Input: part model. Units: mm. Frame: model coordinates. A direction names the side the tool comes from. Give positions to 0.01 mm unless a question says otherwise; leave off trailing zeros. Write each loop counter-clockwise with the first axis right and the second up, starting at its lowest first coordinate (ties: lowest second). Pieces come first, ordered by that corner, then holes.
```python
from build123d import *

# Parameters (mm, degrees)
SKETCH1_W           = 50
SKETCH1_H           = 58
BOSS_EXTRUDE1_DEPTH = 3
SKETCH2_W           = 50
SKETCH2_H           = 3
BOSS_EXTRUDE2_DEPTH = 20
SKETCH6_R           = 3
BOSS_EXTRUDE3_DEPTH = 25
SKETCH7_R           = 6
CUT_EXTRUDE2_DEPTH  = 24
SKETCH9_R           = 1.9
CUT_EXTRUDE3_DEPTH  = 4
SKETCH10_R          = 1.25
CUT_EXTRUDE4_DEPTH  = 10
BOSS_EXTRUDE4_REACH = 31.5
SKETCH11_R          = 4.5
SKETCH12_R          = 3
SKETCH12_R_2        = 2.25
CUT_EXTRUDE5_DEPTH  = 1


with BuildPart() as part:
    # Sketch1 → Boss-Extrude1 (new body)
    with BuildSketch(Plane.XY):
        with Locations((-30.619684785, 7.512687188)):
            Rectangle(SKETCH1_W, SKETCH1_H)
    extrude(amount=BOSS_EXTRUDE1_DEPTH)

    # Sketch2 → Boss-Extrude2 (add)
    with BuildSketch(Plane(origin=(0, 0, 0), x_dir=(-1, 0, 0), z_dir=(0, 0, -1))):
        with Locations((30.619684785, -19.987312812)):
            Rectangle(SKETCH2_W, SKETCH2_H)
    extrude(amount=BOSS_EXTRUDE2_DEPTH)

    # Sketch6 → Boss-Extrude3 (add)
    with BuildSketch(Plane.XY.offset(3)):
        with Locations((-30.619684785, -1.487312812)):
            Circle(SKETCH6_R)
    extrude(amount=BOSS_EXTRUDE3_DEPTH)

    # Sketch7 → Cut-Extrude2 (cut, through all)
    with BuildSketch(Plane.XY.offset(3)):
        with Locations((-30.619684785, 21.012687188)):
            Circle(SKETCH7_R)
    extrude(amount=-CUT_EXTRUDE2_DEPTH, mode=Mode.SUBTRACT)

    # Sketch9 → Cut-Extrude3 (cut, through all)
    with BuildSketch(Plane(origin=(0, -18.487312812, 0), x_dir=(1, 0, 0), z_dir=(0, 1, 0))):
        with Locations((-18.119684785, 10)):
            Circle(SKETCH9_R)
        with Locations((-43.119684785, 10)):
            Circle(SKETCH9_R)
    extrude(amount=-CUT_EXTRUDE3_DEPTH, mode=Mode.SUBTRACT)

    # Sketch10 → Cut-Extrude4 (cut)
    with BuildSketch(Plane.XY.offset(3)):
        with Locations((-40.145964226, 26.512687188)):
            Circle(SKETCH10_R)
        with Locations((-21.093405343, 26.512687188)):
            Circle(SKETCH10_R)
        with Locations((-30.619684785, 10.012687188)):
            Circle(SKETCH10_R)
    extrude(amount=-CUT_EXTRUDE4_DEPTH, mode=Mode.SUBTRACT)

    # Sketch11 → Boss-Extrude4 (add, up to next)
    with BuildSketch(Plane.XY.offset(9.5), mode=Mode.PRIVATE) as boss_extrude4_sk1:
        with Locations((-30.619684785, -1.487312812)):
            Circle(SKETCH11_R)
    boss_extrude4_tool1 = extrude(boss_extrude4_sk1.sketch, amount=-BOSS_EXTRUDE4_REACH, mode=Mode.PRIVATE) - part.part
    add(boss_extrude4_tool1.solids().sort_by_distance((-30.619685, -1.487313, 9.5))[0])

    # Sketch12 → Cut-Extrude5 (cut)
    with BuildSketch(Plane.XY.offset(21.5)):
        with Locations((-30.619684785, -1.487312812)):
            Circle(SKETCH12_R)
        with Locations((-30.619684785, -1.487312812)):
            Circle(SKETCH12_R_2, mode=Mode.SUBTRACT)
    extrude(amount=CUT_EXTRUDE5_DEPTH, mode=Mode.SUBTRACT)


solid = part.part
```
Q1. Pin query (flat end, axial travel): pin 1 (1 mm diameter, centred on x = -45, y = 20, fed in from +Z); pin 2 (3 mm diameter, centred on x = -21.09, y = 26.51, fed in from -Z); pin 3 (4.5 mm diameter, centred on x = -18.12, z = -10, fed in from +Y). Return the tip coordinate at first contact, or that it passes through.
Q2. Material intervals for line 1 along X through (y, z) = (-20, -10); line 2 along Z through (x, y) = (-31.5, 1.5); line 3 along Z through (x, y) = (-13, 32.5), sorted ascending.
Q3. Section A-A, the plane z = -10. Return the cut outline in (x, y), then the cut area to 3 significant figures.
Q4. Section D-D, the plane z = -16.5. Return the cut outline in (x, y).
Q5. Section B-B, the plane y = 19. Return the cut outline in (x, z).
Q6. Section C-C, the plane z = 15. Return the cut outline in (x, y), then the cut area to 3 significant figures.
Q7. Access query for faces 1 (the flat face through (-31, 3, 0)), 2 (the flat face through (-30, 1, 21.5)), 3 (the cylindrical face through (-27.85, -2.64, 25.21)). Directions: +Z, -Z, +X, -X, +Y, -Y. A direction counts if a zero-diameter tool reaches every point of the face in a straight line with its end or side. Return the directions, or none.
Q8. Mould query, pull axis Z, two halves, no side actions, for faces 4 (the flat face through (-55.62, 3, 1)), 5 (the cylindrical face through (-17.243, -19.966, -8.314)), 6 (the flat face through (-30, -20, -20)), 7 (the cylindrical face through (-45.02, -19.97, -10.08)). Classes: +Z half, -Z half, draft (parallel to the pull), parting line (faces both ways), or undercut.
Solutions:
1. pin 1: stops at z = 3
1. pin 2: stops at z = 0
1. pin 3: stops at y = -18.49
2. line 1: x = -55.62 to -45.02, -41.22 to -20.02, -16.22 to -5.62
2. line 2: z = 0 to 9.5
2. line 3: z = 0 to 3
3. outline: (-55.62, -21.49) - (-45.02, -21.49) - (-45.02, -18.49) - (-55.62, -18.49) - close; (-41.22, -21.49) - (-20.02, -21.49) - (-20.02, -18.49) - (-41.22, -18.49) - close; (-16.22, -21.49) - (-5.62, -21.49) - (-5.62, -18.49) - (-16.22, -18.49) - close
3. area: 127 mm2
4. outline: (-55.62, -21.49) - (-5.62, -21.49) - (-5.62, -18.49) - (-55.62, -18.49) - close
5. outline: (-55.62, 0) - (-36.27, 0) - (-36.27, 3) - (-55.62, 3) - close; (-24.97, 0) - (-5.62, 0) - (-5.62, 3) - (-24.97, 3) - close
6. outline: circle Ø6 at (-30.62, -1.49)
6. area: 28.3 mm2
7. face 1: -Z, +X, -X, +Y
7. face 2: none
7. face 3: +Z
8. face 4: draft
8. face 5: undercut
8. face 6: -Z half
8. face 7: undercut
